Study the drawing (mm; zero at the part's minimum x, y, z) and answer. A direction names the side the tool comes from. Round coordinates to 2 decimals unless told otherwise and drop trailing zeros. Order: outer loops, then holes, each group sorted by start corner. A loop starts at its lowest first (then second) coordinate and runs counter-clockwise, first axis right, second up. Notation, with made-up numbers: (18.25, -6) -> (48.25, -6) arc R4 ccw to (48.25, -2) -> close; hole circle Ø10 at (-35, -0.5). An arc over 180 degrees is marked (long way). Answer in a Markdown table with one row per item. Add a question column.
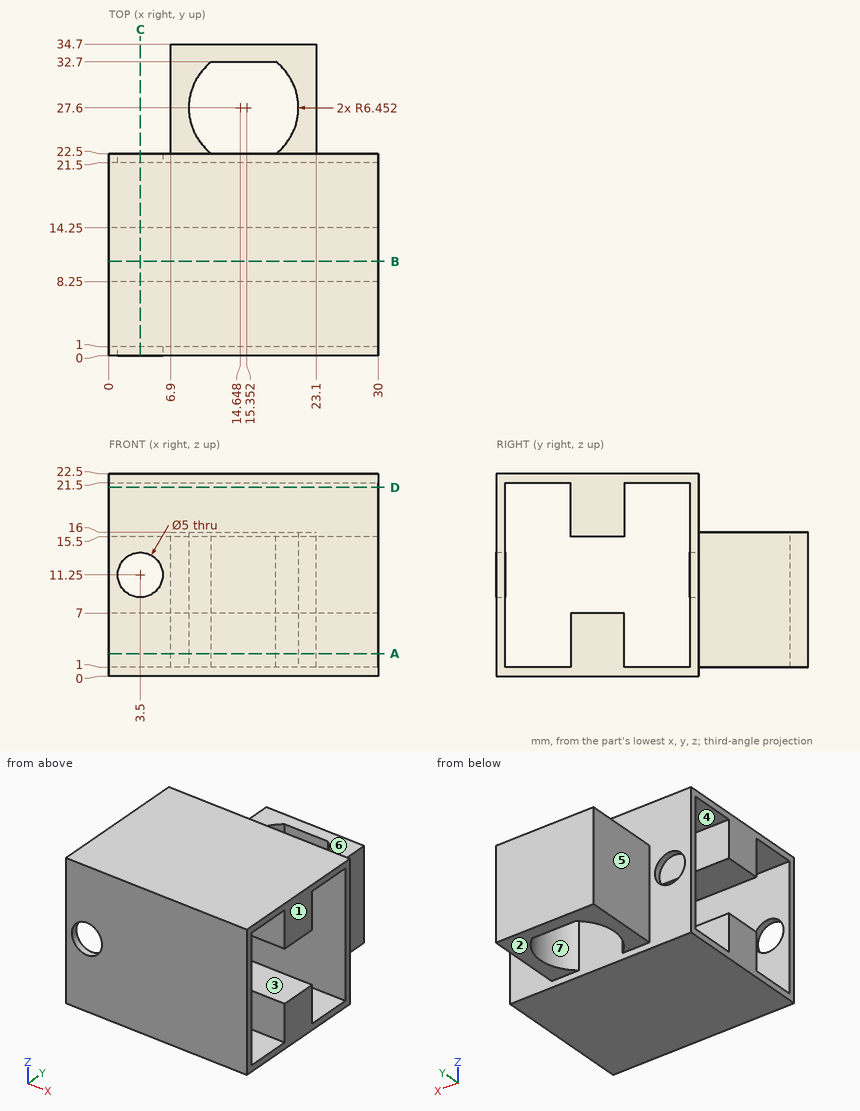
Item 1: The part is cut by section C-C, the plane x = 3.5. Give the vertices of the cut face in (y, z).
Item 2: Flat-ended cylindrical pins translate along their axes: P1, Ø3, axis at x = 13, z = 19.5, coming from the +Y side; P2, Ø12, axis at x = 4.5, y = 30, coming from the -Z side; P3, Ø6, axis at x = 12, y = 26, coming from the +Z side. Find the tip coordinate at first contact, or state that the pin passes through.
Item 3: The part is cut by section D-D, the plane z = 21. Give the vertices of the cut face in (x, y), and give its area (3 significant figures).
Item 4: A tool of negligible diameter and unlimited length cuts with its end or side. For the marked faces 4, 5, 6 and 7, from which of +Z, -Z, +X, -X, +Y, -Y can it reach the whole face along a straight path? Write none if from no direction.
Item 5: For a pull along Z with two mould halves and no side action, classify the marked faces 1, 2 and 3 as released by +Z, released by -Z, zero draft, split by the parting line, or undercut.
Item 6: The part is cut by section A-A, the plane z = 2.5. Give the vertices of the cut face in (x, y), and give its area (3 significant figures).
Item 7: Find the intervals of material crossed by probe 1 along Y at (x, z) = (14.5, 6.25); probe 2 along Y at (x, z) = (1.5, 3.25); probe 3 along Z at (x, y) = (3.5, 0.6), in increasing order. Write a range as [from, to].
Item 8: The part is cut by section B-B, the plane y = 10.5. Give the vertices of the cut face in (x, z), and give its area (3 significant figures).
Resolved:
| question | item | result |
|---|---|---|
| 1 | outline | (0, 0) -> (22.5, 0) -> (22.5, 8.75) -> (21.5, 8.75) -> (21.5, 1) -> (14.25, 1) -> (14.25, 7) -> (8.25, 7) -> (8.25, 1) -> (1, 1) -> (1, 8.75) -> (0, 8.75) -> close; (0, 13.75) -> (1, 13.75) -> (1, 21.5) -> (8.25, 21.5) -> (8.25, 15.5) -> (14.25, 15.5) -> (14.25, 21.5) -> (21.5, 21.5) -> (21.5, 13.75) -> (22.5, 13.75) -> (22.5, 22.5) -> (0, 22.5) -> close |
| 2 | P1 | y = 22.5 |
| 2 | P2 | z = 1 |
| 2 | P3 | z = 16 |
| 3 | outline | (0, 0) -> (30, 0) -> (30, 1) -> (0, 1) -> close; (0, 8.25) -> (30, 8.25) -> (30, 14.25) -> (0, 14.25) -> close; (0, 21.5) -> (30, 21.5) -> (30, 22.5) -> (0, 22.5) -> close |
| 3 | area | 240 mm2 |
| 4 | face 4 | +X, -X |
| 4 | face 5 | +Z, -Z, -X, +Y |
| 4 | face 6 | +Z, +X, -X, +Y |
| 4 | face 7 | +Z, -Z |
| 5 | face 1 | zero draft |
| 5 | face 2 | released by -Z |
| 5 | face 3 | undercut |
| 6 | outline | (0, 0) -> (30, 0) -> (30, 1) -> (0, 1) -> close; (0, 8.25) -> (30, 8.25) -> (30, 14.25) -> (0, 14.25) -> close; (0, 21.5) -> (30, 21.5) -> (30, 22.5) -> (23.1, 22.5) -> (23.1, 34.7) -> (6.9, 34.7) -> (6.9, 22.5) -> (0, 22.5) -> close; hole (11.4, 22.5) -> (18.6, 22.5) arc R6.45 ccw to (18.6, 32.7) -> (11.4, 32.7) arc R6.45 ccw to start |
| 6 | area | 329 mm2 |
| 7 | probe 1 | [0, 1], [8.25, 14.25], [21.5, 22.5], [32.7, 34.7] |
| 7 | probe 2 | [0, 1], [8.25, 14.25], [21.5, 22.5] |
| 7 | probe 3 | [0, 8.75], [13.75, 22.5] |
| 8 | outline | (0, 0) -> (30, 0) -> (30, 7) -> (0, 7) -> close; (0, 15.5) -> (30, 15.5) -> (30, 22.5) -> (0, 22.5) -> close |
| 8 | area | 420 mm2 |
